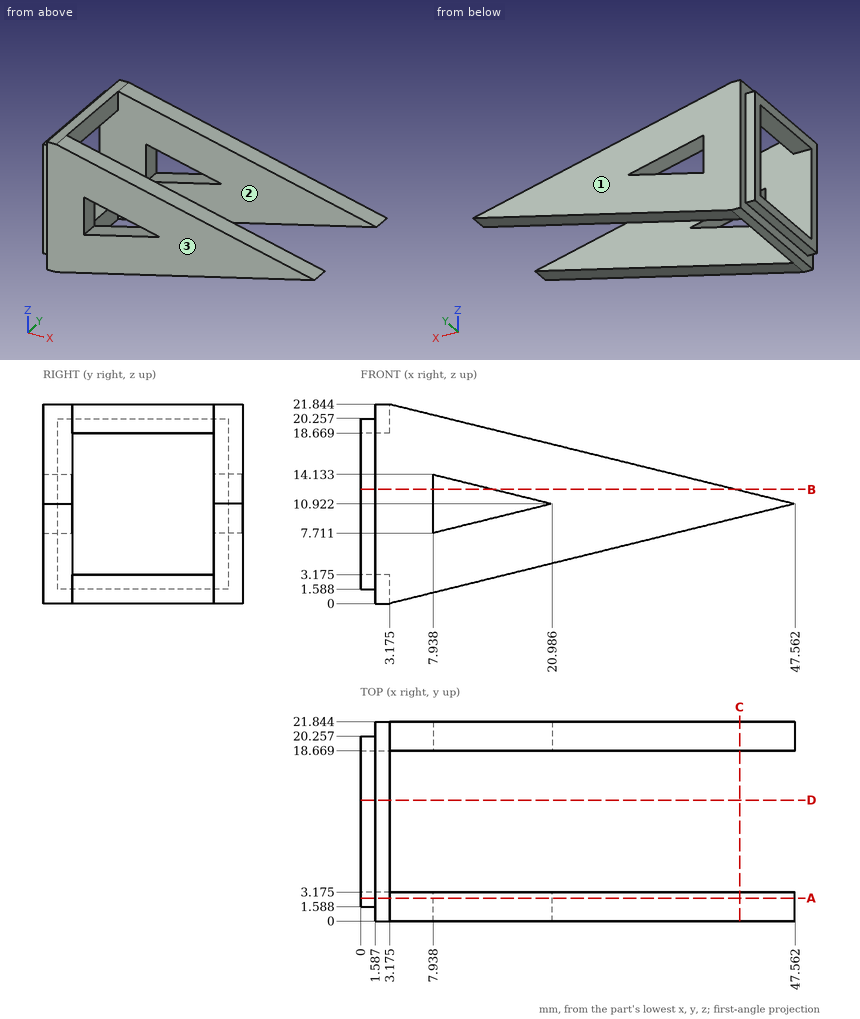
Check sheet for the drawn part. Datum: minimum x, y, z corner. Units: mm. Coordinates: 2 decimals unless noted, no trailing zeros. Loops run counter-clockwise (first coordinate to the right, second up) from the corner with the lowest first, then second, coordinate; pieces in that order, holes last. Notation, with made-up numbers: M -19,68.25 L 31,68.25 A10 ccw 31,73.25 Z; hole C -14.75,2.5 d1. An arc over 180 degrees is marked long. Answer as a JSON object with one key per item and string values.
1. Scan lines: L1, parallel to Y at x = 2.5, z = 8.5 (1 decimal); L2, parallel to X at y = 16.5, z = 19.5 (1 decimal); L3, parallel to Z at x = 25, y = 19.25 (1 decimal). Record each from-to range of solid material in increasing order. Write a range as from..to.
Outcome:
{"L1": "0..3.2, 18.7..21.8", "L2": "0..3.2", "L3": "5.4..16.5"}
2. Sectioned sample at A-A on y = 2.5. Record the cut outline in (x, z) (1 decimal), and give its area (3 significant figures).
Outcome:
{"outline": "M 0,1.6 L 1.6,1.6 L 1.6,0 L 3.2,0 L 47.6,10.9 L 3.2,21.8 L 1.6,21.8 L 1.6,20.3 L 0,20.3 Z; hole M 7.9,7.7 L 21,10.9 L 7.9,14.1 Z", "area": "507 mm²"}
3. Release check for a two-part mould opening along Y. For the marked faces 1, 2 and 3 record: pulls with the +Y half, pulls with the -Y half, needs draft (parallel to the pull), parting line crosses it, or undercut.
Outcome:
{"face 1": "pulls with the +Y half", "face 2": "undercut", "face 3": "pulls with the -Y half"}
4. Sectioned sample at D-D on y = 13.25. Record the cut outline in (x, z) (1 decimal), and give its area (3 significant figures).
Outcome:
{"outline": "M 0,1.6 L 1.6,1.6 L 1.6,0 L 3.2,0 L 3.2,3.2 L 0,3.2 Z; M 0,18.7 L 3.2,18.7 L 3.2,21.8 L 1.6,21.8 L 1.6,20.3 L 0,20.3 Z", "area": "15.1 mm²"}
5. Depth check by flat-ended pin: P1, Ø1.7, axis at x = 0.5, y = 6.5, coming from the -Z side; P2, Ø1, axis at y = 9, z = 1, coming from the +X side (1 decimal); P3, Ø12, axis at x = 29.5, y = 3, coming from the +Z side. Enter the tip coordinate at first touch or a pass-through.
Outcome:
{"P1": "z = 1.59", "P2": "x = 3.2", "P3": "z = 16.84"}
6. Sectioned sample at B-B on z = 12.5. Record the cut outline in (x, y) (1 decimal), and give its area (3 significant figures).
Outcome:
{"outline": "M 0,1.6 L 1.6,1.6 L 1.6,0 L 7.9,0 L 7.9,3.2 L 0,3.2 Z; M 0,18.7 L 7.9,18.7 L 7.9,21.8 L 1.6,21.8 L 1.6,20.3 L 0,20.3 Z; M 14.6,0 L 41.1,0 L 41.1,3.2 L 14.6,3.2 Z; M 14.6,18.7 L 41.1,18.7 L 41.1,21.8 L 14.6,21.8 Z", "area": "214 mm²"}
7. Sectioned sample at C-C on x = 41.5. Record the cut outline in (y, z) (1 decimal).
Outcome:
{"outline": "M 0,9.4 L 3.2,9.4 L 3.2,12.4 L 0,12.4 Z; M 18.7,9.4 L 21.8,9.4 L 21.8,12.4 L 18.7,12.4 Z"}
